Source: CAD feature listing. Evaluate the final solid. Frame: model axes, mm. Face numbers are marked on the shaded views. A direction names the side the tool comes from. Round coordinates to 2 decimals unless told otherwise and drop trailing zeros. Loops run counter-clockwise (first coordinate to the right, second up) from the corner with the lowest first, then second, coordinate; pieces in that order, holes last. Notation, with made-up numbers: (-4.75, 77) - (54.25, 77) arc R17 ccw to (54.25, 103) - close; hole circle Ø7 at (-8.75, -12). An arc over 180 degrees is marked (long way). One line per question, with ' | ' between items.
from build123d import *

# Parameters (mm, degrees)
F0_W     = 28.390645
F0_H     = 79.825648
F0_W_2   = 21.75387
F0_H_2   = 18.066776
F1_DEPTH = 25.4


with BuildPart() as f1:
    # F0 (on Top) → F1 (new body)
    with BuildSketch(Plane.XY):
        Polygon((-39.636292, 47.194839), (-14.379677, 47.194839), (14.010968, 47.194839), (47.563549, 47.194839), (47.563549, 66.183388), (-39.636292, 66.183388), align=None)
        with Locations((-0.184354, 7.282015)):
            Rectangle(F0_W, F0_H)
        with BuildLine():
            Line((14.010968, -32.630809), (-14.379677, -32.630809))
            Line((-14.379677, -32.630809), (-14.564033, -32.630809))
            Line((-14.564033, -32.630809), (-14.564033, -42.790807))
            ThreePointArc((-14.564033, -42.790807), (-10.844289, -51.771063), (-1.864033, -55.490807))
            Line((-1.864033, -55.490807), (14.010968, -55.490807))
            Line((14.010968, -55.490807), (14.010968, -32.630809))
        make_face()
        with BuildLine():
            Line((33.92129, -32.630809), (14.010968, -32.630809))
            Line((14.010968, -32.630809), (14.010968, -55.490807))
            Line((14.010968, -55.490807), (42.97516, -55.490807))
            ThreePointArc((42.97516, -55.490807), (51.955416, -51.771063), (55.67516, -42.790807))
            Line((55.67516, -42.790807), (55.67516, -32.630809))
            Line((55.67516, -32.630809), (33.92129, -32.630809))
        make_face()
        with Locations((44.798225, -23.597421)):
            Rectangle(F0_W_2, F0_H_2)
    extrude(amount=F1_DEPTH)


solid = f1.part
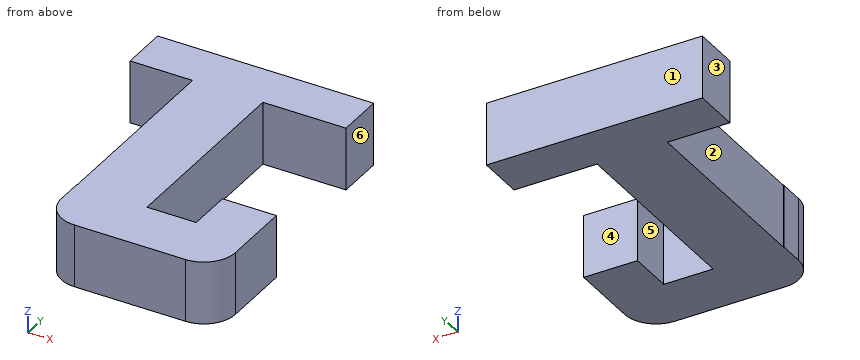
1. Contact query for flat-ended pins moving along their axis: P1, Ø3, axis at y = -37.5, z = 17, coming from the -X side; P2, Ø5.5, axis at y = -24, z = 10.5, coming from the -X side; P3, Ø5, axis at x = -19, y = 16.5, coming from the -Z side; P4, Ø1, axis at x = -20, z = 5.5, coming from the -Y side. Output: stop coordinate, or through.
Worked out:
P1: stops at x = -14.56 | P2: stops at x = -14.38 | P3: passes through | P4: stops at y = 47.19
2. Material intervals for probe 1 along Y at (x, z) = (31.5, 5.75); probe 2 along Y at (x, z) = (36.5, 3.25); probe 3 along X at (y, z) = (-17, 11.25), sorted ascending.
Worked out:
probe 1: y = -55.49 to -32.63, 47.19 to 66.18 | probe 2: y = -55.49 to -14.56, 47.19 to 66.18 | probe 3: x = -14.38 to 14.01, 33.92 to 55.68
3. Section query A-A, the plane y = -31. Return loops of the section in (x, z).
Worked out:
outline: (-14.38, 0) - (14.01, 0) - (14.01, 25.4) - (-14.38, 25.4) - close; (33.92, 0) - (55.68, 0) - (55.68, 25.4) - (33.92, 25.4) - close
4. Section query B-B, the plane x = 29. Return loops of the section in (y, z), plus the area to 3 significant figures.
Worked out:
outline: (-55.49, 0) - (-32.63, 0) - (-32.63, 25.4) - (-55.49, 25.4) - close; (47.19, 0) - (66.18, 0) - (66.18, 25.4) - (47.19, 25.4) - close | area: 1,060 mm2
5. Section query D-D, the plane y = 20. Return loops of the section in (x, z), plus the area to 3 significant figures.
Worked out:
outline: (-14.38, 0) - (14.01, 0) - (14.01, 25.4) - (-14.38, 25.4) - close | area: 721 mm2
6. Access query for the marked faces 4, 5 and 6. Directions: +Z, -Z, +X, -X, +Y, -Y. A direction counts if a zero-diameter tool reaches every point of the face in a straight line with its end or side. Return the directions, or none.
Worked out:
face 4: +Z, -Z, +X | face 5: +Z, -Z | face 6: +Z, -Z, +X, +Y
7. Mould query, pull axis Y, two halves, no side actions, for the marked faces 1, 2 and 3. Classes: released by +Y, released by -Y, zero draft, split by the parting line, or undercut.
Worked out:
face 1: released by +Y | face 2: undercut | face 3: zero draft
8. Section query C-C, the plane z = 11.75. Return loops of the section in (x, y).
Worked out:
outline: (-39.64, 47.19) - (-14.38, 47.19) - (-14.38, -32.63) - (-14.56, -32.63) - (-14.56, -42.79) arc R12.7 ccw to (-1.86, -55.49) - (42.98, -55.49) arc R12.7 ccw to (55.68, -42.79) - (55.68, -14.56) - (33.92, -14.56) - (33.92, -32.63) - (14.01, -32.63) - (14.01, 47.19) - (47.56, 47.19) - (47.56, 66.18) - (-39.64, 66.18) - close
